Read the model definition and answer for the solid it produces. Units are mm, in the model's axes. A direction names the side the tool comes from. Coordinates: 2 decimals unless noted, no trailing zeros. Write each loop counter-clockwise with the first axis right and the second up, starting at its lowest first coordinate (ties: lowest second). Pieces come first, ordered by that corner, then holes. Notation, with made-up numbers: (13, -13) - (50, -13) arc R23 ccw to (50, 23) - close; hole circle Ø7 at (18, 14). An arc over 180 degrees is marked (long way). Return JSON: item names as keys, results as strings.
```python
from build123d import *

# Parameters (mm, degrees)
F0_W      = 85
F0_H      = 23
F0_H_2    = 40
F1_DEPTH  = 3
F2_W      = 3
F2_H      = 23
F3_DEPTH  = 24
F4_W      = 3
F4_H      = 23
F5_DEPTH  = 25
F6_R      = 4
F7_DEPTH  = 200
F8_R      = 2.096138
F9_DEPTH  = 101.9
F10_R     = 2.08537
F11_DEPTH = 136.8


with BuildPart() as f1:
    # F0 (on Top) → F1 (new body)
    with BuildSketch(Plane.XY):
        with Locations((42.5, 11.5)):
            Rectangle(F0_W, F0_H)
        with Locations((42.5, -20)):
            Rectangle(F0_W, F0_H_2)
    extrude(amount=F1_DEPTH)

    # F2 (on face) → F3 (join)
    with BuildSketch(Plane.XY.offset(3)):
        with Locations((1.5, 11.5)):
            Rectangle(F2_W, F2_H)
        with Locations((83.5, 11.5)):
            Rectangle(F2_W, F2_H)
    extrude(amount=F3_DEPTH)

    # F4 (on face) → F5 (join)
    with BuildSketch(Plane.XY.offset(27)):
        with Locations((1.5, 11.5)):
            Rectangle(F4_W, F4_H)
    extrude(amount=F5_DEPTH)

    # F6 (on face) → F7 (cut)
    with BuildSketch(Plane.YZ.offset(85)):
        with Locations((11.5, 13.5)):
            Circle(F6_R)
    extrude(amount=-F7_DEPTH, mode=Mode.SUBTRACT)

    # F8 (on Right) → F9 (cut)
    with BuildSketch(Plane.YZ):
        with Locations((19.000002, 13.309989)):
            Circle(F8_R)
    extrude(amount=F9_DEPTH, mode=Mode.SUBTRACT)

    # F10 (on Right) → F11 (cut)
    with BuildSketch(Plane.YZ):
        with Locations((4, 12.777778)):
            Circle(F10_R)
    extrude(amount=F11_DEPTH, mode=Mode.SUBTRACT)


solid = f1.part
```
(1) Flat-ended cylindrical pins translate along their axes: P1, Ø3.5, axis at x = 2, z = 31, coming from the -Y side; P2, Ø2.5, axis at x = 83.5, y = 8.5, coming from the +Z side; P3, Ø1, axis at y = 4, z = 30, coming from the +X side. Find the tip coordinate at first contact, or state that the pin passes through.
Answer:
{"P1": "y = 0", "P2": "z = 27", "P3": "x = 3"}
(2) Determine the mould class of faces 4 (the face through (83, 12, 27)), 5 (the face through (1, 0, 27)), 6 (the face through (1.479, 4.962, 10.928)) for opening direction Z: +Z half, -Z half, draft (parallel to the pull), parting line (faces both ways), or undercut.
Answer:
{"face 4": "+Z half", "face 5": "draft", "face 6": "undercut"}
(3) Straight lines are drawn through the part: line 1 (Z direction, x = 83, y = 4); line 2 (X direction, y = 11, z = 23.5); line 3 (Z direction, x = 15.5, y = 1). For each, find the intervals that lie inside material, in ascending order. Write a range as from..to.
Answer:
{"line 1": "0..10.69, 14.86..27", "line 2": "0..3, 82..85", "line 3": "0..3"}
(4) A cutting plane is placed at A-A (y = 4). Determine the outline of the cut face in (x, z).
Answer:
{"outline": "(0, 0) - (85, 0) - (85, 10.69) - (82, 10.69) - (82, 3) - (3, 3) - (3, 10.69) - (0, 10.69) - close; (0, 14.86) - (3, 14.86) - (3, 52) - (0, 52) - close; (82, 14.86) - (85, 14.86) - (85, 27) - (82, 27) - close"}
(5) Which of the six approach directions +Z, -Z, +X, -X, +Y, -Y give full straight-line access (tool end or side, diameter ignored) to faces 1 (the face through (3, 11, 27)), 2 (the face through (83, 0, 15)), 3 (the face through (1.479, 16.906, 13.402))?
Answer:
{"face 1": "+Z, +Y, -Y", "face 2": "+Z, +X, -X, -Y", "face 3": "+X, -X"}
(6) A cutting plane is placed at B-B (z = 20.5). Determine the outline of the cut face in (x, y).
Answer:
{"outline": "(0, 0) - (3, 0) - (3, 23) - (0, 23) - close; (82, 0) - (85, 0) - (85, 23) - (82, 23) - close"}
(7) A cutting plane is placed at C-C (y = 11.5). Determine the outline of the cut face in (x, z), and give its area (3 significant figures).
Answer:
{"outline": "(0, 0) - (85, 0) - (85, 9.5) - (82, 9.5) - (82, 3) - (3, 3) - (3, 9.5) - (0, 9.5) - close; (0, 17.5) - (3, 17.5) - (3, 52) - (0, 52) - close; (82, 17.5) - (85, 17.5) - (85, 27) - (82, 27) - close", "area": "426 mm²"}
(8) A cutting plane is placed at D-D (x = 73.5). Determine the outline of the cut face in (y, z).
Answer:
{"outline": "(-40, 0) - (23, 0) - (23, 3) - (-40, 3) - close"}
